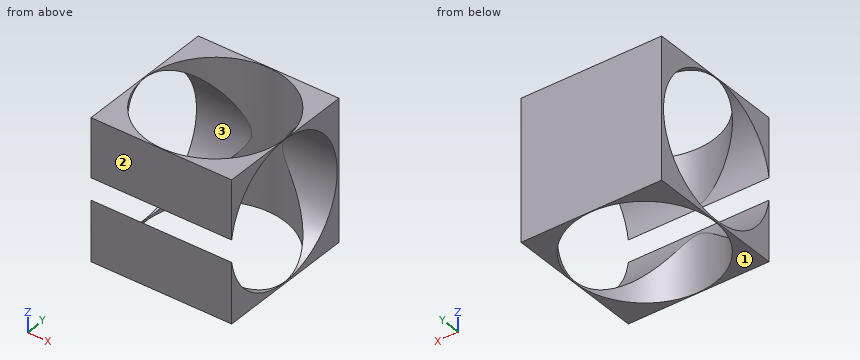
from build123d import *

# Parameters (mm, degrees)
F0_W     = 76.2
F0_H     = 76.2
F1_DEPTH = 76.2
F2_R     = 37.756667
F3_DEPTH = 76.2
F5_DEPTH = 78.74


with BuildPart() as f1:
    # F0 (on Front) → F1 (new body)
    with BuildSketch(Plane.XZ):
        with Locations((38.1, -38.1)):
            Rectangle(F0_W, F0_H)
    extrude(amount=F1_DEPTH)

    # F2 (on face) → F3 (cut)
    with BuildSketch(Plane.XY):
        with Locations((38.248464, -38.1)):
            Circle(F2_R)
    extrude(amount=-F3_DEPTH, mode=Mode.SUBTRACT)

    # F4 (on face) → F5 (cut)
    with BuildSketch(Plane(origin=(0, 0, 0), x_dir=(0, -1, 0), z_dir=(-1, 0, 0))):
        with BuildLine():
            Line((76.2, -43.645483), (76.2, -31.788889))
            ThreePointArc((76.2, -31.788889), (1.288281, -37.717186), (76.2, -43.645483))
        make_face()
    extrude(amount=-F5_DEPTH, mode=Mode.SUBTRACT)


solid = f1.part
Model file for the job. Use its own axes, mm. Face numbers are marked on the shaded views. Give positions to 0.01 mm unless a question says otherwise; leave off trailing zeros. Order: outer loops, then holes, each group sorted by start corner. A loop starts at its lowest first (then second) coordinate and runs counter-clockwise, first axis right, second up. Notation, with made-up numbers: (-1.5, 86) - (49.5, 86) arc R34 cw to (49.5, 116) - close; hole circle Ø4 at (-13.5, 4). An arc over 180 degrees is marked (long way). Write item = value, one per line. Start each with the question number.
1. Probe line 1 along Y through (x, z) = (24, -27.5); line 2 along Z through (x, y) = (8, -9); line 3 along Y through (x, z) = (59.5, -47.5). List the from-to ranges inside material, lowest first.
2. Cut at B-B, the plane y = -53.5. List the corners of the cut face in (x, z), and give its area (3 significant figures).
3. Two-plate mould, pull along Z, no slides. Class the marked faces 1, 2 and 3: pulls with the +Z half, pulls with the -Z half, needs draft (parallel to the pull), parting line crosses it, or undercut.
4. Cut at C-C, the plane z = -68. List the corners of the cut face in (x, y), and give its area (3 significant figures).
5. Cut at D-D, the plane x = 66. List the corners of the cut face in (y, z), and give its area (3 significant figures).
6. Cut at A-A, the plane x = 16. List the corners of the cut face in (y, z), and give its area (3 significant figures).
Taken from the geometry:
q1.line_1 = -76.2 to -75.26, -2.7 to 0
q1.line_2 = -76.2 to -60.56, -14.87 to 0
q1.line_3 = -76.2 to -75.38, -2.58 to 0
q2.outline = (0, -76.2) - (3.78, -76.2) - (3.78, -72.5) - (0, -72.5) - close; (0, -2.94) - (3.78, -2.94) - (3.78, 0) - (0, 0) - close; (72.72, -76.2) - (76.2, -76.2) - (76.2, -72.5) - (72.72, -72.5) - close; (72.72, -2.94) - (76.2, -2.94) - (76.2, 0) - (72.72, 0) - close
q2.area = 48.2 mm²
q3.face_1 = pulls with the -Z half
q3.face_2 = needs draft
q3.face_3 = undercut
q4.outline = (0, -76.2) - (76.2, -76.2) - (76.2, -61.42) - (67.94, -61.42) arc R37.76 cw to (8.55, -61.42) - (0, -61.42) - close; (0, -16.54) - (7.25, -16.54) arc R37.76 cw to (69.24, -16.54) - (76.2, -16.54) - (76.2, 0) - (0, 0) - close
q4.area = 1,080 mm²
q5.outline = (-76.2, -76.2) - (-63.7, -76.2) - (-63.7, -66.17) arc R37.69 cw to (-76.2, -43.65) - close; (-76.2, -31.79) arc R37.69 cw to (-63.7, -9.27) - (-63.7, 0) - (-76.2, 0) - close; (-12.5, -76.2) - (0, -76.2) - (0, 0) - (-12.5, 0) - (-12.5, -10.9) arc R37.69 cw to (-12.5, -64.54) - close
q5.area = 982 mm²
q6.outline = (-76.2, -76.2) - (-68.61, -76.2) - (-68.61, -61.02) arc R37.69 cw to (-76.2, -43.65) - close; (-76.2, -31.79) arc R37.69 cw to (-68.61, -14.42) - (-68.61, 0) - (-76.2, 0) - close; (-7.59, -76.2) - (0, -76.2) - (0, 0) - (-7.59, 0) - (-7.59, -16.85) arc R37.69 cw to (-7.59, -58.59) - close
q6.area = 726 mm²
